Verification items for the finished model (mm, model axes). A direction names the side the tool comes from. Give positions to 0.01 mm unless a question says otherwise; leave off trailing zeros. Loops run counter-clockwise (first coordinate to the right, second up) from the corner with the lowest first, then second, coordinate; pieces in that order, holes last. Notation, with made-up numbers: M -33,25.25 L -28,25.25 A21 cw -28,57.25 Z; hole C 45,17.25 d7. An arc over 180 degrees is marked long. Put each result on its own line as item: value. Start each with the question number.
from build123d import *

# Parameters (mm, degrees)
SKETCH1_R           = 25
BOSS_EXTRUDE1_DEPTH = 60
SKETCH2_W           = 14
SKETCH2_H           = 10
CUT_EXTRUDE1_DEPTH  = 80


with BuildPart() as part:
    # Sketch1 → Boss-Extrude1 (new, symmetric)
    with BuildSketch(Plane.XY):
        Circle(SKETCH1_R)
    extrude(amount=BOSS_EXTRUDE1_DEPTH, both=True)

    # Sketch2 → Cut-Extrude1 (cut)
    with BuildSketch(Plane.XY.offset(60)):
        with Locations((0, 25)):
            Rectangle(SKETCH2_W, SKETCH2_H)
    extrude(amount=-CUT_EXTRUDE1_DEPTH, mode=Mode.SUBTRACT)


solid = part.part
Q1. Go/stop test with flat-tipped pins: pin 1 (4.5 mm diameter, centred on y = 23, z = 37, fed in from +X); pin 2 (4 mm diameter, centred on x = 2.5, z = 18.5, fed in from +Y); pin 3 (3 mm diameter, centred on y = 20, z = 4.5, fed in from -X). Record where each tip stops, or that it passes through.
Q2. Cross-section at D-D, the plane z = -35. Record the boundary of the cut face in (x, y).
Q3. Set-up check for faces 1 (the face through (0, 23, -20)), 2 (the face through (0, 0, 60)): record each of +Z, -Z, +X, -X, +Y, -Y from which the full face is reachable in a straight line by a thin tool's end or side.
Q4. Cross-section at C-C, the plane y = 15. Record the boundary of the cut face in (x, z).
Q5. Release check for a two-part mould opening along X. For faces 3 (the face through (11.5, -22.2, 0.8)), 4 (the face through (0, 20, 21)), 5 (the face through (0, 0, -60)) record: pulls with the +X half, pulls with the -X half, needs draft (parallel to the pull), parting line crosses it, or undercut.
Q6. Cross-section at A-A, the plane x = 0. Record the boundary of the cut face in (y, z).
Q7. Cross-section at B-B, the plane z = 41.5. Record the boundary of the cut face in (x, y), then the cut area to 3 significant figures.
Q8. Scan lines: L1, parallel to Z at x = -5, y = 22.5; L2, parallel to Y at x = -0.5, z = -33.5 (3 decimals); L3, parallel to Y at x = -15, z = 4. Record each from-to range of solid material in increasing order.
Ans:
1. pin 1: stops at x = 13.94
1. pin 2: stops at y = 20
1. pin 3: stops at x = -16.82
2. outline: C 0,0 d50
3. face 1: +Z, +Y
3. face 2: +Z, +X, -X, +Y, -Y
4. outline: M -20,-60 L 20,-60 L 20,60 L -20,60 Z
5. face 3: parting line crosses it
5. face 4: undercut
5. face 5: needs draft
6. outline: M -25,-60 L 25,-60 L 25,-20 L 20,-20 L 20,60 L -25,60 Z
7. outline: M -7,20 L -7,24 A25 ccw long 7,24 L 7,20 Z
7. area: 1,900 mm^2
8. L1: z = -60 to -20
8. L2: y = -24.995 to 24.995
8. L3: y = -20 to 20
